```python
from build123d import *

# Parameters (mm, degrees)
SKETCH1_R           = 7.5
BOSS_EXTRUDE1_DEPTH = 25
SKETCH2_R           = 10
BOSS_EXTRUDE2_DEPTH = 5
SKETCH3_R           = 1.5
CUT_EXTRUDE1_DEPTH  = 5
CHAMFER1_SIZE       = 2


with BuildPart() as part:
    # Sketch1 → Boss-Extrude1 (new body)
    with BuildSketch(Plane.XY):
        Circle(SKETCH1_R)
    extrude(amount=BOSS_EXTRUDE1_DEPTH)

    # Sketch2 → Boss-Extrude2 (add)
    with BuildSketch(Plane.XY.offset(25)):
        Circle(SKETCH2_R)
    extrude(amount=BOSS_EXTRUDE2_DEPTH)

    # Sketch3 → Cut-Extrude1 (cut)
    with BuildSketch(Plane(origin=(0, 0, 0), x_dir=(-1, 0, 0), z_dir=(0, 0, -1))):
        Circle(SKETCH3_R)
    extrude(amount=-CUT_EXTRUDE1_DEPTH, mode=Mode.SUBTRACT)

    # Chamfer1
    chamfer1_edges = [part.edges().sort_by_distance(p)[0] for p in [
        (-10, 0, 30),
    ]]
    chamfer(chamfer1_edges, length=CHAMFER1_SIZE)


solid = part.part
```
For this review, take the finished solid that the model builds, in its own axes (mm). A direction names the side the tool comes from. Coordinates: 2 decimals unless noted, no trailing zeros. Write each loop counter-clockwise with the first axis right and the second up, starting at its lowest first coordinate (ties: lowest second). Pieces come first, ordered by that corner, then holes. Notation, with made-up numbers: (58, -21.5) - (63, -21.5) arc R30 ccw to (63, 6.5) - close; hole circle Ø5 at (-25.75, 82). An arc over 180 degrees is marked (long way). Answer in a Markdown table with one row per item. Add a question column.
Q1. We need section C-C, the plane z = 18. State the section outline as (x, y) points.
Q2. For P1, Ø6, axis at x = -5.5, z = 7.5, coming from the -Y side; P2, Ø1.5, axis at x = 0, y = -0.5, coming from the -Z side; P3, Ø4, axis at x = -6, z = 8, coming from the -Y side, all flat-tipped, find the tip position at first contact; note any pin that passes through.
Q3. We need section A-A, the plane y = 0. State the section outline as (x, z) points, and give its area (3 significant figures).
Q4. For probe 1 along Y at (x, z) = (0, 3); probe 2 along Y at (x, z) = (-1.5, 10); probe 3 along Z at (x, y) = (-8, -4), list the stretches that pass through material, from the lowest coordinate up.
Q5. Tool access review of faces 1 (the flat face through (2, 0, 0)), 2 (the cylindrical face through (1.5, 0.07, 2.46)): name each direction out of +Z, -Z, +X, -X, +Y, -Y from which nothing blocks a thin tool from reaching the whole face with its end or side.
Q6. We need section D-D, the plane z = 2.25. State the section outline as (x, y) points, and give its area (3 significant figures).
Q7. Draft analysis for pull direction X (two halves, no side actions). For faces 3 (the flat face through (0, 0, 30)), 4 (the cylindrical face through (-7.493, 0.33, 12.325)), 5 (the flat face through (0, 0, 5)), state which applies: +X half, -X half, draft (parallel to the pull), parting line (faces both ways), or undercut.
Answer list:
| question | item | result |
|---|---|---|
| 1 | outline | circle Ø15 at (0, 0) |
| 2 | P1 | stops at y = -7.07 |
| 2 | P2 | stops at z = 5 |
| 2 | P3 | stops at y = -6.34 |
| 3 | outline | (-10, 25) - (-7.5, 25) - (-7.5, 0) - (-1.5, 0) - (-1.5, 5) - (1.5, 5) - (1.5, 0) - (7.5, 0) - (7.5, 25) - (10, 25) - (10, 28) - (8, 30) - (-8, 30) - (-10, 28) - close |
| 3 | area | 456 mm2 |
| 4 | probe 1 | y = -7.5 to -1.5, 1.5 to 7.5 |
| 4 | probe 2 | y = -7.35 to 7.35 |
| 4 | probe 3 | z = 25 to 29.06 |
| 5 | face 1 | -Z, +X, -X, +Y, -Y |
| 5 | face 2 | -Z |
| 6 | outline | circle Ø15 at (0, 0); hole circle Ø3 at (0, 0) |
| 6 | area | 170 mm2 |
| 7 | face 3 | draft |
| 7 | face 4 | parting line |
| 7 | face 5 | undercut |
